Read the model definition and answer for the solid it produces. Units are mm, in the model's axes. A direction names the side the tool comes from. Round coordinates to 2 decimals unless told otherwise and drop trailing zeros. Order: outer loops, then holes, each group sorted by start corner. A loop starts at its lowest first (then second) coordinate and runs counter-clockwise, first axis right, second up. Notation, with made-up numbers: (-27, 19.5) -> (-23, 19.5) arc R12 ccw to (-23, 41.5) -> close; hole circle Ø10 at (22.5, -4). An arc over 180 degrees is marked (long way). One line per item, written item: value. Start each with the question number.
1. Section D-D (z = 12) is taken. Give the vertices of the cut face in (x, y).
2. Section C-C (y = 0.5) is taken. Give the vertices of the cut face in (x, z), then the cut area to 3 significant figures.
3. Section A-A (z = 0) is taken. Give the vertices of the cut face in (x, y), then the cut area to 3 significant figures.
4. Section B-B (x = 0) is taken. Give the vertices of the cut face in (y, z), then the cut area to 3 significant figures.
5. Consider line 1 (X direction, y = 0.5, z = 0); line 2 (X direction, y = 0.4, z = -1); line 3 (X direction, y = 1.5, z = -6). Determine where each line is inside the solid, lowest interval first.
6. For faces 1 (the face through (-4, 1, 18.8)), 2 (the face through (-3, 2, 3)), 3 (the face through (-3.15, 0.99, 16.45)), 4 (the face through (6, 1, 15)), 5 (the face through (-6, 1, 15)), determine the directions among +Z, -Z, +X, -X, +Y, -Y from which every point of the face is accessible in a straight line to the end or side of a thin tool.
7. A flat-ended cylindrical pin translates along its axis: pin 1 Ø1 at (x, y) = (-1.5, 1) entering from +Z. Find the tip coordinate at first contact, or state that the pin passes through.
from build123d import *

# Parameters (mm, degrees)
SKETCH1_R           = 3
BOSS_EXTRUDE1_DEPTH = 2
SKETCH2_R           = 12.5
SKETCH2_R_2         = 3
BOSS_EXTRUDE2_DEPTH = 2
SKETCH4_W           = 12
SKETCH4_H           = 0.2
CUT_EXTRUDE1_DEPTH  = 4
FILLET3_R           = 0.35
FILLET4_R           = 0.15


with BuildPart() as part:
    # Sketch1 → Boss-Extrude1 (new body)
    with BuildSketch(Plane(origin=(0, 0, 0), x_dir=(1, 0, 0), z_dir=(0, 1, 0))):
        Polygon((-6, 6), (-6, -13.291502622), (-6, -19), (-2.70227506, -19), (-3.619175359, -13.8), (0, -13.8), (3.619175359, -13.8), (2.70227506, -19), (6, -19), (6, -13.291502622), (6, 6), align=None)
        with Locations(Location((0, 0, 0), (0, 0, 270))):
            Circle(SKETCH1_R, mode=Mode.SUBTRACT)
    extrude(amount=BOSS_EXTRUDE1_DEPTH)

    # Sketch2 → Boss-Extrude2 (add)
    with BuildSketch(Plane(origin=(0, 0, 0), x_dir=(1, 0, 0), z_dir=(0, 1, 0))):
        Circle(SKETCH2_R)
        with Locations(Location((0, 0, 0), (0, 0, 270))):
            Circle(SKETCH2_R_2, mode=Mode.SUBTRACT)
    extrude(amount=BOSS_EXTRUDE2_DEPTH)

    # Sketch4 → Cut-Extrude1 (cut)
    with BuildSketch(Plane(origin=(0, 2, 0), x_dir=(1, 0, 0), z_dir=(0, 1, 0))):
        with Locations((0, -18.9)):
            Rectangle(SKETCH4_W, SKETCH4_H)
    extrude(amount=-CUT_EXTRUDE1_DEPTH, mode=Mode.SUBTRACT)

    # Fillet3
    fillet3_edges = [part.edges().sort_by_distance(p)[0] for p in [
        (3.619175359, 1, 13.8),
        (-3.619175359, 1, 13.8),
    ]]
    fillet(fillet3_edges, radius=FILLET3_R)

    # Fillet4
    fillet4_edges = [part.edges().sort_by_distance(p)[0] for p in [
        (2.737540456, 1, 18.8),
        (-2.737540456, 1, 18.8),
    ]]
    fillet(fillet4_edges, radius=FILLET4_R)


solid = part.part
Answer:
1. outline: (-6, 0) -> (6, 0) -> (6, 2) -> (-6, 2) -> close
2. outline: (-6, 10.97) arc R12.5 ccw (long way) to (6, 10.97) -> (6, 18.8) -> (2.92, 18.8) arc R0.15 ccw to (2.77, 18.62) -> (3.55, 14.21) arc R0.35 cw to (3.2, 13.8) -> (-3.2, 13.8) arc R0.35 cw to (-3.55, 14.21) -> (-2.77, 18.62) arc R0.15 ccw to (-2.92, 18.8) -> (-6, 18.8) -> close; hole circle Ø6 at (0, 0)
2. area: 512 mm^2
3. outline: (-12.5, 0) -> (-3, 0) -> (-3, 2) -> (-12.5, 2) -> close; (3, 0) -> (12.5, 0) -> (12.5, 2) -> (3, 2) -> close
3. area: 38.0 mm^2
4. outline: (0, -12.5) -> (2, -12.5) -> (2, -3) -> (0, -3) -> close; (0, 3) -> (2, 3) -> (2, 13.8) -> (0, 13.8) -> close
4. area: 40.6 mm^2
5. line 1: -12.5 to -3, 3 to 12.5
5. line 2: -12.46 to -2.83, 2.83 to 12.46
5. line 3: -10.97 to 10.97
6. face 1: +Z, +X, -X, +Y, -Y
6. face 2: +Z, -Z, +X, -X, +Y
6. face 3: +Y, -Y
6. face 4: +Z, +X, +Y, -Y
6. face 5: +Z, -X, +Y, -Y
7. pin 1: z = 13.8
